The drawing under review shows one solid part. Ordinate dimensions are in mm from its lowest x, y, z. Round coordinates to 2 decimals unless told otherwise and drop trailing zeros. Order: outer loops, then holes, each group sorted by start corner. A loop starts at its lowest first (then second) coordinate and runs counter-clockwise, first axis right, second up. Notation, with made-up numbers: M 7.5,51 L 58.5,51 A29 cw 58.5,80 Z; hole C 35,56.5 d5. An arc over 180 degrees is marked long. Answer as a JSON object with one key per item and string values. Group by question number.
1. Add section C-C on z = 20. State the section outline as (x, y) points.
2. Add section D-D on y = 11.75. State the section outline as (x, z) points.
3. To check wall thickness, follow probe 1 along Y at (x, z) = (4.5, 8); probe 2 along Z at (x, y) = (30.5, 8.5); probe 3 along Z at (x, y) = (12, 8.75). State the ranges of each line that lie inside material, in increasing order. Write a range as [from, to].
4. Add section A-A on x = 20. State the section outline as (y, z) points.
5. Clearance check with flat-ended pins moving along their axes: P1, Ø8, axis at x = 28.5, z = 21.5, coming from the -Y side; P2, Ø2.5, axis at x = 20, y = 18.5, coming from the -Z side; P3, Ø2, axis at x = 13.5, z = 30.5, coming from the +Y side; P4, Ø6, axis at x = 33.5, y = 2.5, coming from the +Z side. State where each tip first meets the part, or that it passes through.
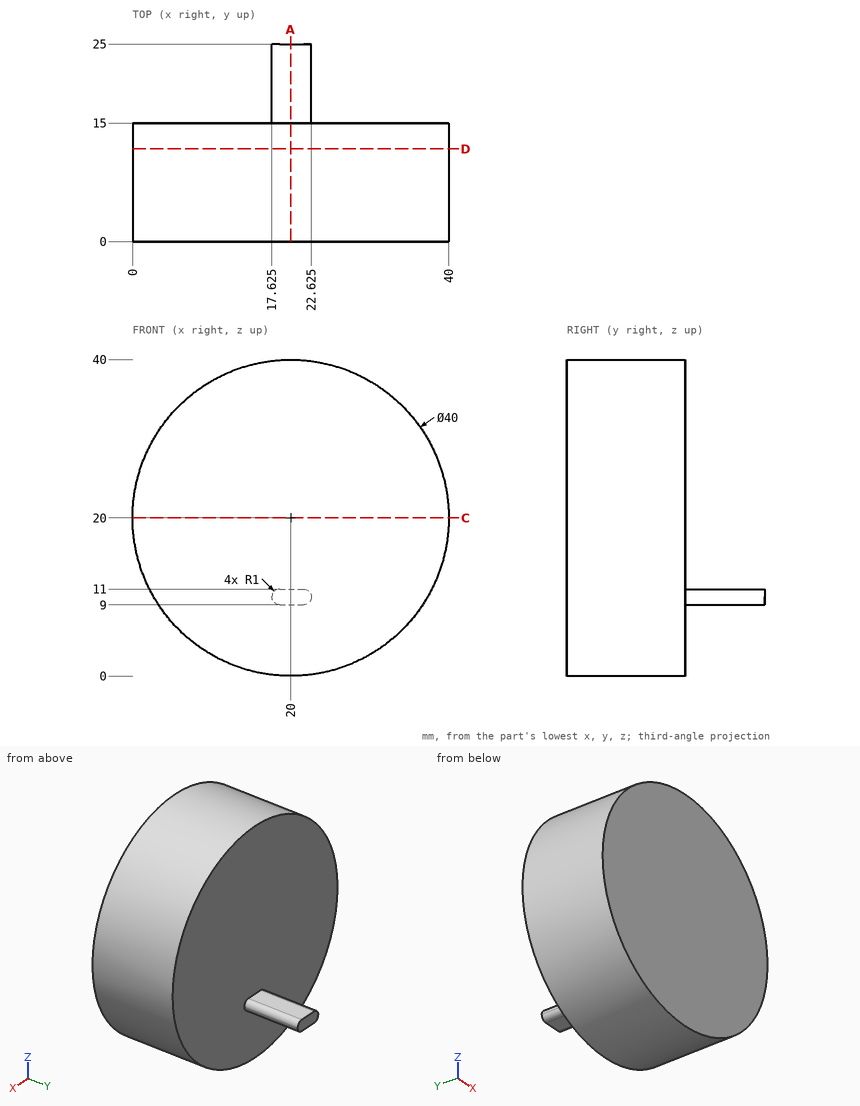
Recorded:
{
 "1": {"outline": "M 0,0 L 40,0 L 40,15 L 0,15 Z"},
 "2": {"outline": "C 20,20 d40"},
 "3": {"probe 1": "y = [0, 15]", "probe 2": "z = [2.98, 37.02]", "probe 3": "z = [1.67, 38.33]"},
 "4": {"outline": "M 0,0 L 15,0 L 15,9 L 25,9 L 25,11 L 15,11 L 15,40 L 0,40 Z"},
 "5": {"P1": "stops at y = 0", "P2": "stops at z = 9", "P3": "stops at y = 15", "P4": "stops at z = 37.02"}
}
